from build123d import *

# Parameters (mm, degrees)
MAIN_SHAPE_DEPTH        = 0.6
TABS_DEPTH              = 154.060061459
TABS_DEPTH_BACK         = 154.060061459
CHIN_GUARD_DEPTH        = 0.6
FILLET1_R               = 20
CUT_EXTRUDE1_DEPTH      = 172.662513141
CUT_EXTRUDE1_DEPTH_BACK = 172.662513141
CUT_EXTRUDE2_DEPTH      = 172.662513141
CUT_EXTRUDE2_DEPTH_BACK = 172.662513141


with BuildPart() as part:
    # Sketch1 → Main Shape (new body)
    with BuildSketch(Plane.XY):
        with BuildLine():
            Line((-24, -91.764766734), (24, -91.764766734))
            Line((24, -91.764766734), (78.266232563, -84.05670244))
            ThreePointArc((78.266232563, -84.05670244), (97.655491519, -79.289252293), (115.711102551, -70.764766734))
            ThreePointArc((115.711102551, -70.764766734), (120.685143325, -65.658407438), (122.5, -58.764766734))
            ThreePointArc((122.5, -58.764766734), (120.227482046, -43.118277124), (113.597722286, -28.764766734))
            ThreePointArc((113.597722286, -28.764766734), (107.811505455, -22.955172168), (100.180351554, -19.955641477))
            Line((100.180351554, -19.955641477), (60.74391922, -13.264766734))
            ThreePointArc((60.74391922, -13.264766734), (50.804108255, -9.246591688), (43.461443341, -1.434367632))
            ThreePointArc((43.461443341, -1.434367632), (36.448172688, 5.805997675), (26.941855461, 9.15842781))
            Line((26.941855461, 9.15842781), (17, 10.235233266))
            Line((17, 10.235233266), (10, 0))
            Line((10, 0), (-10, 0))
            Line((-10, 0), (-17, 10.235233266))
            Line((-17, 10.235233266), (-26.941855461, 9.15842781))
            ThreePointArc((-26.941855461, 9.15842781), (-36.448172688, 5.805997675), (-43.461443341, -1.434367632))
            ThreePointArc((-43.461443341, -1.434367632), (-50.804108255, -9.246591688), (-60.74391922, -13.264766734))
            Line((-60.74391922, -13.264766734), (-100.180351554, -19.955641477))
            ThreePointArc((-100.180351554, -19.955641477), (-107.811505455, -22.955172168), (-113.597722286, -28.764766734))
            ThreePointArc((-113.597722286, -28.764766734), (-120.227482046, -43.118277124), (-122.5, -58.764766734))
            ThreePointArc((-122.5, -58.764766734), (-120.685143325, -65.658407438), (-115.711102551, -70.764766734))
            ThreePointArc((-115.711102551, -70.764766734), (-97.655491519, -79.289252293), (-78.266232563, -84.05670244))
            Line((-78.266232563, -84.05670244), (-24, -91.764766734))
        make_face()
    extrude(amount=MAIN_SHAPE_DEPTH)

    # Sketch2 → Tabs (cut, two sides: drawn at the far end of the back side and taken through both)
    with BuildSketch(Plane.XY.offset(0.6).offset(-TABS_DEPTH_BACK)):
        with BuildLine():
            Line((-121, -58.764766734), (-121, -56.764766734))
            Line((-121, -56.764766734), (-115.742268041, -53.771413729))
            ThreePointArc((-115.742268041, -53.771413729), (-113.511139955, -43.427720083), (-109.089826236, -33.814088314))
            Line((-109.089826236, -33.814088314), (-111.5, -28.264766734))
            Line((-111.5, -28.264766734), (-110.3, -26.664766734))
            Line((-110.3, -26.664766734), (-108.3, -25.664766734))
            Line((-108.3, -25.664766734), (-106.7, -26.864766734))
            Line((-106.7, -26.864766734), (-107.9, -28.464766734))
            Line((-107.9, -28.464766734), (-106.3, -29.664766734))
            Line((-106.3, -29.664766734), (-98.84870892, -19.729711961))
            Line((-98.84870892, -19.729711961), (-100.180351554, -19.955641477))
            ThreePointArc((-100.180351554, -19.955641477), (-107.811505455, -22.955172168), (-113.597722286, -28.764766734))
            ThreePointArc((-113.597722286, -28.764766734), (-120.227482046, -43.118277124), (-122.5, -58.764766734))
            ThreePointArc((-122.5, -58.764766734), (-120.767844146, -65.510135516), (-116, -70.586357152))
            Line((-116, -70.586357152), (-116, -58.764766734))
            Line((-116, -58.764766734), (-118, -58.764766734))
            Line((-118, -58.764766734), (-118, -60.764766734))
            Line((-118, -60.764766734), (-120, -60.764766734))
            Line((-120, -60.764766734), (-121, -58.764766734))
        make_face()
        with BuildLine():
            Line((110.3, -26.664766734), (111.5, -28.264766734))
            Line((111.5, -28.264766734), (109.089826236, -33.814088314))
            ThreePointArc((109.089826236, -33.814088314), (113.511139955, -43.427720083), (115.742268041, -53.771413729))
            Line((115.742268041, -53.771413729), (121, -56.764766734))
            Line((121, -56.764766734), (121, -58.764766734))
            Line((121, -58.764766734), (120, -60.764766734))
            Line((120, -60.764766734), (118, -60.764766734))
            Line((118, -60.764766734), (118, -58.764766734))
            Line((118, -58.764766734), (116, -58.764766734))
            Line((116, -58.764766734), (116, -70.586357152))
            ThreePointArc((116, -70.586357152), (120.767844146, -65.510135516), (122.5, -58.764766734))
            ThreePointArc((122.5, -58.764766734), (120.227482046, -43.118277124), (113.597722286, -28.764766734))
            ThreePointArc((113.597722286, -28.764766734), (107.811505455, -22.955172168), (100.180351554, -19.955641477))
            Line((100.180351554, -19.955641477), (98.84870892, -19.729711961))
            Line((98.84870892, -19.729711961), (106.3, -29.664766734))
            Line((106.3, -29.664766734), (107.9, -28.464766734))
            Line((107.9, -28.464766734), (106.7, -26.864766734))
            Line((106.7, -26.864766734), (108.3, -25.664766734))
            Line((108.3, -25.664766734), (110.3, -26.664766734))
        make_face()
    extrude(amount=TABS_DEPTH + TABS_DEPTH_BACK, mode=Mode.SUBTRACT)

    # Sketch5 → Chin guard (add)
    with BuildSketch(Plane.XY.offset(0.6)):
        Polygon((-78.266232563, -84.05670244), (-24, -121.764766734), (24, -121.764766734), (78.266232563, -84.05670244), (24, -91.764766734), (-24, -91.764766734), align=None)
    extrude(amount=-CHIN_GUARD_DEPTH)

    # Fillet1
    fillet1_edges = [part.edges().sort_by_distance(p)[0] for p in [
        (-24, -121.764766734, 0.3),
        (24, -121.764766734, 0.3),
        (78.266232563, -84.05670244, 0.3),
        (-78.266232563, -84.05670244, 0.3),
    ]]
    fillet(fillet1_edges, radius=FILLET1_R)

    # Sketch6 → Cut-Extrude1 (cut, two sides: drawn at the far end of the back side and taken through both)
    with BuildSketch(Plane.XY.offset(0.6).offset(-CUT_EXTRUDE1_DEPTH_BACK)):
        with BuildLine():
            Line((-60.74391922, -13.264766734), (-60.74391922, 16.735233266))
            Line((-60.74391922, 16.735233266), (60.74391922, 16.735233266))
            Line((60.74391922, 16.735233266), (60.74391922, -13.264766734))
            ThreePointArc((60.74391922, -13.264766734), (0, -8.148349205), (-60.74391922, -13.264766734))
        make_face()
    extrude(amount=CUT_EXTRUDE1_DEPTH + CUT_EXTRUDE1_DEPTH_BACK, mode=Mode.SUBTRACT)

    # Sketch7 → Cut-Extrude2 (cut, two sides: drawn at the far end of the back side and taken through both)
    with BuildSketch(Plane.XY.offset(0.6).offset(-CUT_EXTRUDE2_DEPTH_BACK)):
        with BuildLine():
            Line((-109.089826236, -33.814088314), (-102.449085801, -38.79464364))
            ThreePointArc((-102.449085801, -38.79464364), (-101.786812206, -41.123983791), (-103.854832759, -42.384032539))
            Line((-103.854832759, -42.384032539), (-112.807082802, -41.45817123))
            ThreePointArc((-112.807082802, -41.45817123), (-111.116237814, -37.554538094), (-109.089826236, -33.814088314))
        make_face()
        with BuildLine():
            Line((103.854832759, -42.384032539), (112.807082802, -41.45817123))
            ThreePointArc((112.807082802, -41.45817123), (111.116237814, -37.554538094), (109.089826236, -33.814088314))
            Line((109.089826236, -33.814088314), (102.449085801, -38.79464364))
            ThreePointArc((102.449085801, -38.79464364), (101.786812206, -41.123983791), (103.854832759, -42.384032539))
        make_face()
    extrude(amount=CUT_EXTRUDE2_DEPTH + CUT_EXTRUDE2_DEPTH_BACK, mode=Mode.SUBTRACT)


solid = part.part
Can you work these out from the model? Positions are in its coordinate system, mm. A direction names the side the tool comes from. Coordinates: 2 decimals unless noted, no trailing zeros. Order: outer loops, then holes, each group sorted by start corner. A loop starts at its lowest first (then second) coordinate and runs counter-clockwise, first axis right, second up. Notation, with made-up numbers: (-0.75, 53) - (47.25, 53) arc R33 cw to (47.25, 82) - close; hole circle Ø9 at (-22.5, 42.5). An arc over 180 degrees is marked (long way). Answer as a JSON object with one key per item and string values. Group by question number.
Q1. I need wall thicknesses on line 1 (Y direction, x = -104, z = 0.4); line 2 (Y direction, x = -102.5, z = 0.3); line 3 (X direction, y = -61, z = 0.3). Which ranges of each line are inside material? Lowest first, please. Write a range as from..to.
Q2. Imagine slicing it at A-A (y = -49). Please give me the cut outline in (x, z).
Q3. Imagine slicing it at B-B (x = -69). Please give me the cut outline in (y, z), and give its area (3 significant figures).
Q4. On a 3-axis mill with a long thin cutter (end or side, diameter ignored), from which of +Z, -Z, +X, -X, +Y, -Y can I reach the whole of each face in a straight line? I mean faces 4 (the face through (80.06, -16.54, 0.3)), 5 (the face through (105.816, -36.27, 0.296)), 6 (the face through (-102.63, -24.77, 0.3)). Say none if no direction works.
Q5. We'd pull the mould along Y, two halves only. Please class faces 1 (the face through (51.532, -102.633, 0.304)), 2 (the face through (-105.816, -36.27, 0.296)), 3 (the face through (-79.53, -16.452, 0.296)): +Y half, -Y half, draft (parallel to the pull), parting line (faces both ways), or undercut.
Determined:
{
 "1": {"line 1": "y = -76.79..-42.37, -37.63..-26.6", "line 2": "y = -77.43..-42.03, -38.76..-24.6", "line 3": "x = -116..116"},
 "2": {"outline": "(-115.01, 0) - (115.01, 0) - (115.01, 0.6) - (-115.01, 0.6) - close"},
 "3": {"outline": "(-90.5, 0) - (-14.67, 0) - (-14.67, 0.6) - (-90.5, 0.6) - close", "area": "45.5 mm2"},
 "4": {"face 4": "+Z, -Z, +X, +Y", "face 5": "+Z, -Z, +X", "face 6": "+Z, -Z, +Y"},
 "5": {"face 1": "-Y half", "face 2": "undercut", "face 3": "+Y half"}
}
